```python
from build123d import *

# Parameters (mm, degrees)
SKETCH1_R                      = 110
BOSS_EXTRUDE1_DEPTH            = 40
CUT_EXTRUDE1_DEPTH             = 40
FILLET1_R                      = 6
SKETCH3_R                      = 4.25
CUT_EXTRUDE2_DEPTH             = 40
CIRPATTERN1_COUNT              = 7
FILLET1_OF_CIRPATTERN1_R       = 6
SKETCH4_R                      = 16
CUT_EXTRUDE3_DEPTH             = 5
M4_CLEARANCE_HOLE1_D           = 4.5
M4_CLEARANCE_HOLE1_DEPTH       = 13
M4_CLEARANCE_HOLE1_CSINK_D     = 4.55
M4_CLEARANCE_HOLE1_CSINK_ANGLE = 90
M4_CLEARANCE_HOLE1_TIP         = 1.351936393
CUT_EXTRUDE4_DEPTH             = 41
CIRPATTERN2_COUNT              = 8


with BuildPart() as part:
    # Sketch1 → Boss-Extrude1 (new body)
    with BuildSketch(Plane(origin=(0, 0, 0), x_dir=(1, 0, 0), z_dir=(0, 1, 0))):
        Circle(SKETCH1_R)
    extrude(amount=BOSS_EXTRUDE1_DEPTH)

    # Sketch2 → Cut-Extrude1 (cut)
    with BuildSketch(Plane(origin=(0, 40, 0), x_dir=(1, 0, 0), z_dir=(0, 1, 0))):
        with BuildLine():
            ThreePointArc((-9.508910889, 20.391925208), (-4.869891314, 21.96666016), (0, 22.5))
            Line((0, 22.5), (0, 95))
            ThreePointArc((0, 95), (-20.561763324, 92.748120676), (-40.148734865, 86.099239768))
            Line((-40.148734865, 86.099239768), (-9.508910889, 20.391925208))
        make_face()
    cut_extrude1 = extrude(amount=-CUT_EXTRUDE1_DEPTH, mode=Mode.SUBTRACT)

    # Fillet1
    fillet1_edges = [part.edges().sort_by_distance(p)[0] for p in [
        (0, 20, -22.5),
        (-9.508910889, 20, -20.391925208),
        (-40.148734865, 20, -86.099239768),
        (0, 20, -95),
    ]]
    fillet(fillet1_edges, radius=FILLET1_R)

    # Sketch3 → Cut-Extrude2 (cut)
    with BuildSketch(Plane(origin=(0, 40, 0), x_dir=(1, 0, 0), z_dir=(0, 1, 0))):
        Circle(SKETCH3_R)
    extrude(amount=-CUT_EXTRUDE2_DEPTH, mode=Mode.SUBTRACT)

    # CirPattern1: Cut-Extrude1 ×7 about axis
    cirpattern1_axis = Axis((0, 0, 0), (0, 1, 0))
    for i in range(1, CIRPATTERN1_COUNT):
        add(cut_extrude1.rotate(cirpattern1_axis, i * 360 / CIRPATTERN1_COUNT), mode=Mode.SUBTRACT)

    # Fillet1 of CirPattern1
    fillet1_of_cirpattern1_edges = [part.edges().sort_by_distance(p)[0] for p in [
        (-17.591208356, 20, -14.028520542),
        (-21.871758082, 20, -5.279791511),
        (-92.347423014, 20, -22.292453044),
        (-74.273990834, 20, -59.231531177),
        (-21.935878024, 20, 5.006721014),
        (-17.764725337, 20, 13.808132883),
        (-75.006618089, 20, 58.301005505),
        (-92.618151657, 20, 21.139488726),
        (-9.76238413, 20, 20.271799528),
        (-0.280492078, 20, 22.498251581),
        (-1.184299887, 20, 94.992617786),
        (-41.218955216, 20, 85.592042451),
        (9.76238413, 20, 20.271799528),
        (17.414957436, 20, 14.246727958),
        (73.529820285, 20, 60.152851377),
        (41.218955216, 20, 85.592042451),
        (21.935878024, 20, 5.006721014),
        (21.996588801, 20, -4.732872398),
        (92.874486047, 20, -19.983239013),
        (92.618151657, 20, 21.139488726),
        (17.591208356, 20, -14.028520542),
        (10.01434015, 20, -20.148523305),
        (42.282769521, 20, -85.071542842),
        (74.273990834, 20, -59.231531177),
    ]]
    fillet(fillet1_of_cirpattern1_edges, radius=FILLET1_OF_CIRPATTERN1_R)

    # Sketch4 → Cut-Extrude3 (cut)
    with BuildSketch(Plane(origin=(0, 40, 0), x_dir=(1, 0, 0), z_dir=(0, 1, 0))):
        Circle(SKETCH4_R)
    extrude(amount=-CUT_EXTRUDE3_DEPTH, mode=Mode.SUBTRACT)

    # M4 Clearance Hole1
    with Locations(Plane(origin=(0, 35, 0), x_dir=(1, 0, 0), z_dir=(0, 1, 0))):
        with Locations((8, 8), (-8, 8), (-8, -8), (8, -8)):
            CounterSinkHole(M4_CLEARANCE_HOLE1_D / 2, M4_CLEARANCE_HOLE1_CSINK_D / 2, depth=M4_CLEARANCE_HOLE1_DEPTH, counter_sink_angle=M4_CLEARANCE_HOLE1_CSINK_ANGLE)
            with Locations((0, 0, -(M4_CLEARANCE_HOLE1_DEPTH + M4_CLEARANCE_HOLE1_TIP / 2))):  # 118° drill point
                Cone(0, M4_CLEARANCE_HOLE1_D / 2, M4_CLEARANCE_HOLE1_TIP, mode=Mode.SUBTRACT)

    # Sketch10 → Cut-Extrude4 (cut, through all)
    with BuildSketch(Plane(origin=(0, 40, 0), x_dir=(1, 0, 0), z_dir=(0, 1, 0))):
        with BuildLine():
            ThreePointArc((2.060734507, 103.479482862), (4.768805418, 103.390079287), (7.473608029, 103.229817316))
            Line((7.473608029, 103.229817316), (7.942965055, 109.712849321))
            ThreePointArc((7.942965055, 109.712849321), (5.068295614, 109.883176053), (2.190152616, 109.978194346))
            Line((2.190152616, 109.978194346), (2.060734507, 103.479482862))
        make_face()
    cut_extrude4 = extrude(amount=-CUT_EXTRUDE4_DEPTH, mode=Mode.SUBTRACT)

    # CirPattern2: Cut-Extrude4 ×8 about axis
    cirpattern2_axis = Axis((0, 0, 0), (0, 1, 0))
    for i in range(1, CIRPATTERN2_COUNT):
        add(cut_extrude4.rotate(cirpattern2_axis, i * 360 / CIRPATTERN2_COUNT), mode=Mode.SUBTRACT)


solid = part.part
```
Verification items for the finished model (mm, model axes). Coordinates: 2 decimals unless noted, no trailing zeros. Loops run counter-clockwise (first coordinate to the right, second up) from the corner with the lowest first, then second, coordinate; pieces in that order, holes last. Notation, with made-up numbers: (37, 42) - (66, 42) arc R23 ccw to (66, 60) - close; hole circle Ø7 at (29, 46.25). An arc over 180 degrees is marked (long way). Put each result on its own line as item: value.
Item 1: Scan lines: line 1 along Z through (x, y) = (-8, 30.5); line 2 along X through (y, z) = (38, 0); line 3 along X through (y, z) = (34, 44.5). Record each from-to range of solid material in increasing order.
Conclusion:
line 1: z = -109.71 to -94.66, -22.02 to -10.25, -5.75 to 5.75, 10.25 to 21.85, 94.66 to 109.71
line 2: x = -110 to -16, 16 to 22.5, 95 to 110
line 3: x = -100.6 to -83.93, -57.25 to -21.43, -0.55 to 21.43, 54.4 to 100.6
Item 2: Section check C-C (z = -45). Enter the section's corners in (x, y), then the cut area to 3 significant figures.
Conclusion:
outline: (-100.37, 0) - (-83.67, 0) - (-83.67, 40) - (-100.37, 40) - close; (-56.43, 0) - (-20.98, 0) - (-20.98, 40) - (-56.43, 40) - close; (0, 0) - (22.37, 0) - (22.37, 40) - (0, 40) - close; (56.43, 0) - (100.37, 0) - (100.37, 40) - (56.43, 40) - close
area: 4,740 mm2
Item 3: Section check A-A (x = -56). Enter the section's corners in (y, z).
Conclusion:
outline: (0, -94.68) - (40, -94.68) - (40, -44.66) - (0, -44.66) - close; (0, -13.52) - (40, -13.52) - (40, 12.78) - (0, 12.78) - close; (0, 43.53) - (40, 43.53) - (40, 94.68) - (0, 94.68) - close
Item 4: Section check D-D (x = 57.5). Enter the section's corners in (y, z) (3 decimals).
Conclusion:
outline: (0, -93.775) - (40, -93.775) - (40, -75.622) - (0, -75.622) - close; (0, -45.855) - (40, -45.855) - (40, -12.372) - (0, -12.372) - close; (0, 13.124) - (40, 13.124) - (40, 47.039) - (0, 47.039) - close; (0, 75.622) - (40, 75.622) - (40, 93.775) - (0, 93.775) - close
Item 5: Draft check along X on faces 1 (the face through (17.948, 19.72, -16.063)), 2 (the face through (-103.649, 19.72, 36.837)), 3 (the face through (47.24, 19.72, -99.34)). Enter one of: pulls with the +X half, pulls with the -X half, needs draft (parallel to the pull), parting line crosses it, or undercut.
Conclusion:
face 1: undercut
face 2: pulls with the -X half
face 3: pulls with the +X half
Item 6: Gauge pin test, flat ends, axial feed: pin 1 Ø3 at (x, y) = (12, 24.5) entering from -Z; pin 2 Ø6 at (x, y) = (56, 29.5) entering from -Z; pin 3 Ø2 at (y, z) = (22, 83) entering from -X. Record the tip position at first contact, or that the pin passes through.
Conclusion:
pin 1: stops at z = -109.5
pin 2: stops at z = -96.39
pin 3: stops at x = -73.32
Item 7: Section check B-B (y = 31.5). Give the number of separate pieces and of enclosed holes in the cut face, then the cut area to 3 significant figures.
Conclusion:
separate pieces: 1
enclosed holes: 12
area: 24,800 mm2
